Part model, mm, in its own coordinate system. A direction names the side the tool comes from. Round coordinates to 2 decimals unless told otherwise and drop trailing zeros. Write each loop counter-clockwise with the first axis right and the second up, starting at its lowest first coordinate (ties: lowest second). Pieces come first, ordered by that corner, then holes. Notation, with made-up numbers: M -22.75,35.5 L 11.25,35.5 A11 cw 11.25,50.5 Z; hole C 3,77 d11. An arc over 180 degrees is marked long. Use a Markdown table: item, result. Add a question column.
1) Slice it at C-C on y = 1.5. Write the cut outline in (x, z) (3 decimals).
2) Slice it at D-D on z = -22. Write the cut outline in (x, y).
3) Drop flat-ended pins along their axis: P1, Ø6, axis at x = -26, y = 6, coming from the -Z side; P2, Ø4, axis at y = -12, z = -1, coming from the +X side; P3, Ø5, axis at x = 21.5, z = -22, coming from the +Y side; P4, Ø4, axis at y = 17.5, z = 7.5, coming from the +X side. Give the stop position or say it passes through.
4) Two-plate mould, pull along Z, no slides. Class faces 1 (the face through (11, 25.4, 12)), 2 (the face through (3.441, 0.356, -15.497)), 3 (the face through (-5.506, 12.522, -24.796)): released by +Z, released by -Z, zero draft, split by the parting line, or undercut.
5) Wall check: probe 1 along Z at (x, y) = (0, -5.5) (3 decimals); probe 2 along Z at (x, y) = (0, 4.5) (3 decimals); probe 3 along Y at (x, z) = (-27, -5). Give the ranges that are in metal, low to high.
6) Slice it at A-A on x = 0. Write the cut outline in (y, z) (3 decimals), plus the area to 3 significant figures.
7) Slice it at B-B on z = 0. Write the cut outline in (x, y) (3 decimals), plus the area to 3 significant figures.
8) Which spindle directions (+Z, -Z, +X, -X, +Y, -Y) get a long thin tool onto all of the face, cutting with end or side? Do faces 4 (the face through (8, 0, -25)), 5 (the face through (-30.235, -12.522, -23.183)). Say none if no direction does.
```python
from build123d import *

# Parameters (mm, degrees)
F0_R     = 38.1
F3_DEPTH = 25.4
F5_R     = 25.4
F6_DEPTH = 25.4
F8_D     = 31.75


with BuildPart() as f3:
    # F0 (on Front) → F3 (new body)
    with BuildSketch(Plane.XZ):
        Circle(F0_R)
    extrude(amount=F3_DEPTH)

    # F5 (on Front) → F6 (join)
    with BuildSketch(Plane.XZ):
        Circle(F5_R)
    extrude(amount=-F6_DEPTH)

    # F8 (through all)
    with Locations(Plane.XZ.offset(25.4)):
        with Locations((0, 0), (0, 0), (0, 0), (0, 0)):
            Hole(F8_D / 2)


solid = f3.part
```
Entries:
| question | item | result |
|---|---|---|
| 1 | outline | C 0,0 d50.8; hole C 0,0 d31.75 |
| 2 | outline | M -31.11,-25.4 L 31.11,-25.4 L 31.11,0 L 12.69,0 L 12.69,25.4 L -12.69,25.4 L -12.69,0 L -31.11,0 Z |
| 3 | P1 | stops at z = -10.78 |
| 3 | P2 | stops at x = 38.1 |
| 3 | P3 | stops at y = 0 |
| 3 | P4 | stops at x = 24.8 |
| 4 | face 1 | zero draft |
| 4 | face 2 | undercut |
| 4 | face 3 | split by the parting line |
| 5 | probe 1 | z = -38.1 to -15.875, 15.875 to 38.1 |
| 5 | probe 2 | z = -25.4 to -15.875, 15.875 to 25.4 |
| 5 | probe 3 | y = -25.4 to 0 |
| 6 | outline | M -25.4,-38.1 L 0,-38.1 L 0,-25.4 L 25.4,-25.4 L 25.4,-15.875 L -25.4,-15.875 Z; M -25.4,15.875 L 25.4,15.875 L 25.4,25.4 L 0,25.4 L 0,38.1 L -25.4,38.1 Z |
| 6 | area | 1,610 mm^2 |
| 7 | outline | M -38.1,-25.4 L -15.875,-25.4 L -15.875,25.4 L -25.4,25.4 L -25.4,0 L -38.1,0 Z; M 15.875,-25.4 L 38.1,-25.4 L 38.1,0 L 25.4,0 L 25.4,25.4 L 15.875,25.4 Z |
| 7 | area | 1,610 mm^2 |
| 8 | face 4 | +Y |
| 8 | face 5 | +Y, -Y |
